Can you work these out from the drawing? Everything is in mm from the part's minimum corner. Round coordinates to 2 decimals unless told otherwise and drop trailing zeros. Order: outer loops, then holes, each group sorted by start corner. A loop starts at its lowest first (then second) coordinate and runs counter-clockwise, first axis right, second up. Notation, with made-up numbers: (11, 10.5) -> (39, 10.5) arc R6 cw to (39, 17.5) -> close; hole circle Ø10 at (-12, 32). An arc over 180 degrees is marked (long way). One line per item, written item: value.
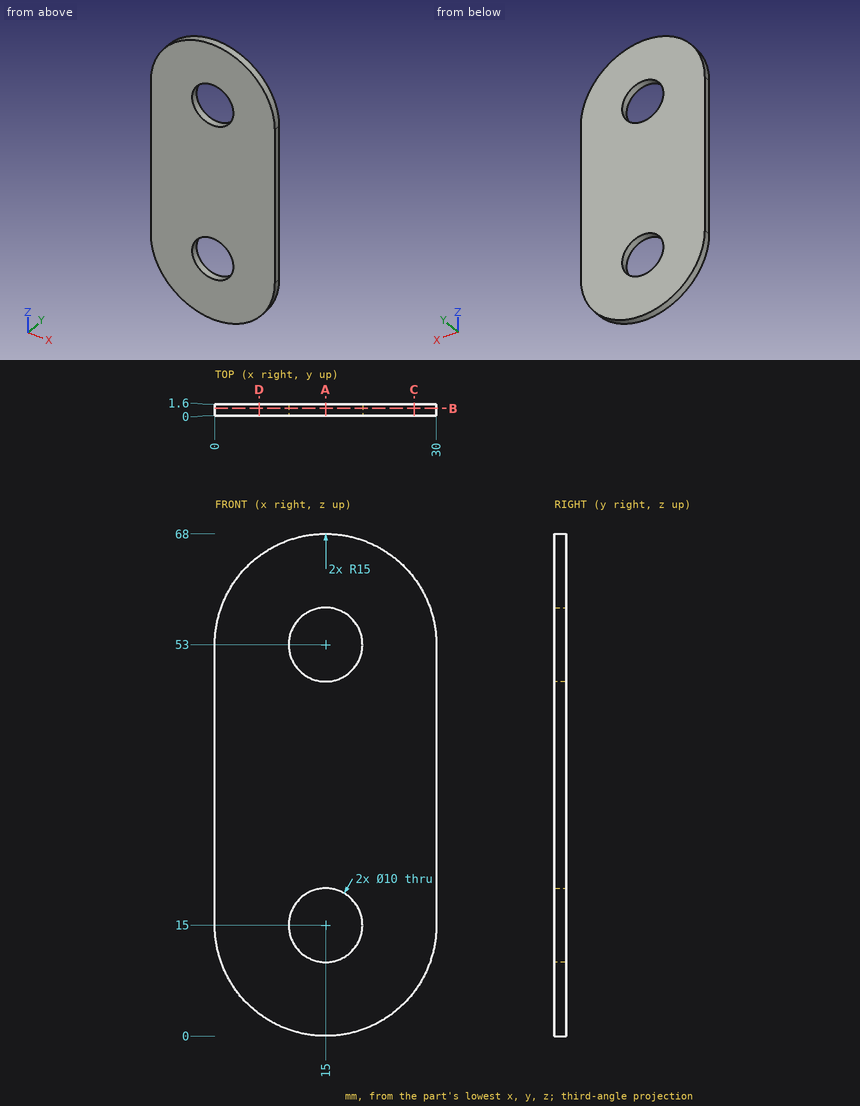
Q1. I want a section at A-A on x = 15. Write out the boundary of the cut face in (y, z), then the cut area to 3 significant figures.
Answers:
outline: (0, 0) -> (1.6, 0) -> (1.6, 10) -> (0, 10) -> close; (0, 20) -> (1.6, 20) -> (1.6, 48) -> (0, 48) -> close; (0, 58) -> (1.6, 58) -> (1.6, 68) -> (0, 68) -> close
area: 76.8 mm2
Q2. I want a section at D-D on x = 6. Write out the boundary of the cut face in (y, z), then the cut area to 3 significant figures.
Answers:
outline: (0, 3) -> (1.6, 3) -> (1.6, 65) -> (0, 65) -> close
area: 99.2 mm2
Q3. I want a section at B-B on y = 1. Write out the boundary of the cut face in (x, z).
Answers:
outline: (0, 15) arc R15 ccw to (30, 15) -> (30, 53) arc R15 ccw to (0, 53) -> close; hole circle Ø10 at (15, 15); hole circle Ø10 at (15, 53)
Q4. I want a section at C-C on x = 27. Write out the boundary of the cut face in (y, z).
Answers:
outline: (0, 6) -> (1.6, 6) -> (1.6, 62) -> (0, 62) -> close
Q5. I need wall thicknesses on line 1 along Z through (x, y) = (15, 0.7); line 2 along X through (y, z) = (1.35, 53); line 3 along Z through (x, y) = (10.5, 0.4). Which ranges of each line are inside material? Lowest first, please.
Answers:
line 1: 0 to 10, 20 to 48, 58 to 68
line 2: 0 to 10, 20 to 30
line 3: 0.69 to 12.82, 17.18 to 50.82, 55.18 to 67.31
Q6. For P1, Ø9, axis at x = 15, z = 53, coming from the +Y side, with a flat end and sliding along its axis, tell me the tip position at first contact or that it passes through.
Answers:
P1: through
